Can you work these out from the model? Positions are in its coordinate system, mm. Round coordinates to 2 decimals unless told otherwise and drop trailing zeros. Order: outer loops, then holes, each group sorted by start corner. A loop starts at its lowest first (then second) coordinate and runs counter-clockwise, first axis right, second up.
Q1. Will these pins go through, and if not, where does the flat tip stop? P1, Ø6, axis at y = -3.5, z = 63.5, coming from the -X side; P2, Ø1.5, axis at x = 0, y = 0, coming from the -Z side (3 decimals); P3, Ø6, axis at x = -5, z = 29, coming from the -Y side; P4, Ø3, axis at x = 4.5, z = 53, coming from the -Y side.
Q2. We'd pull the mould along Y, two halves only. Please class faces 1 (the face through (0.27, -1.22, 36.62)), 2 (the face through (1, -1, -25)), 3 (the face through (-4.16, -3.19, -24.76)): pulls with the +Y half, pulls with the -Y half, needs draft (parallel to the pull), parting line crosses it, or undercut.
Q3. If we section it at A-A (y = 0): Please give me the cut outline in (x, z), plus the area to 3 significant figures.
Q4. If we section it at C-C (z = 19): Please give me the cut outline in (x, y).
Q5. If I drill on line 1 (Y direction, x = 0, z = 62.5); line 2 (Y direction, x = 7, z = 22); line 3 (Y direction, x = 5.25, z = 25), over which ranges is the centre line in solid material (lowest first)?
from build123d import *

# Parameters (mm, degrees)
F0_R          = 10
F1_DEPTH      = 100
F1_DEPTH_BACK = 25
F2_SIZE       = 5
F4_D          = 2.5
F5_SIZE       = 5


with BuildPart() as f1:
    # F0 (on Top) → F1 (new body, two sides)
    with BuildSketch(Plane.XY) as f1_sk:
        Circle(F0_R)
    extrude(amount=F1_DEPTH)
    extrude(f1_sk.sketch, amount=-F1_DEPTH_BACK)

    # F2
    f2_edges = [f1.edges().sort_by_distance(p)[0] for p in [
        (-10, 0, 100),
    ]]
    chamfer(f2_edges, length=F2_SIZE)

    # F4 (through all)
    with Locations(Plane.XY.offset(100)):
        with Locations((0, 0)):
            Hole(F4_D / 2)

    # F5
    f5_edges = [f1.edges().sort_by_distance(p)[0] for p in [
        (-10, 0, -25),
    ]]
    chamfer(f5_edges, length=F5_SIZE)


solid = f1.part
Solution:
1. P1: stops at x = -9.99
1. P2: passes through
1. P3: stops at y = -9.8
1. P4: stops at y = -9.54
2. face 1: undercut
2. face 2: needs draft
2. face 3: parting line crosses it
3. outline: (-10, -20) - (-5, -25) - (-1.25, -25) - (-1.25, 100) - (-5, 100) - (-10, 95) - close; (1.25, -25) - (5, -25) - (10, -20) - (10, 95) - (5, 100) - (1.25, 100) - close
3. area: 2,140 mm2
4. outline: circle Ø20 at (0, 0); hole circle Ø2.5 at (0, 0)
5. line 1: y = -10 to -1.25, 1.25 to 10
5. line 2: y = -7.14 to 7.14
5. line 3: y = -8.51 to 8.51
